Geometry check sheet. Reference: the model listing, model coordinates, mm. Face numbers are marked on the shaded views. Coordinates: 2 decimals unless noted, no trailing zeros. Write each loop counter-clockwise with the first axis right and the second up, starting at its lowest first coordinate (ties: lowest second). Pieces come first, ordered by that corner, then holes. Notation, with made-up numbers: (26, 39.25) -> (34, 39.25) arc R28 ccw to (34, 74.25) -> close; hole circle Ø9 at (36.25, 52.25). An arc over 180 degrees is marked (long way). Answer in a Markdown table with one row per item. Add a question column.
Q1. Release check for a two-part mould opening along Z. For the marked faces 1, 2 and 3 record: pulls with the +Z half, pulls with the -Z half, needs draft (parallel to the pull), parting line crosses it, or undercut.
Q2. Thickness scan on line 1 (Y direction, x = 11, z = -9.75); line 2 (Z direction, x = -8.5, y = -0.5); line 3 (X direction, y = 9.5, z = -3). Record the ranges inside material, lowest first.
Q3. Section check A-A, the plane y = 0. Record the boundary of the cut face in (x, z).
Q4. Gauge pin test, flat ends, axial feed: P1, Ø12, axis at x = 17, y = -5.5, coming from the +Z side; P2, Ø3, axis at y = -3, z = 11.5, coming from the -X side; P3, Ø2, axis at x = -17.5, y = 3, coming from the -Z side. Record the tip position at first contact, or that the pin passes through.
Q5. Section check C-C, the plane x = -15. Record the boundary of the cut face in (y, z).
Q6. Section check B-B, the plane y = 6.75. Record the boundary of the cut face in (x, z), and give its area (3 significant figures).
Q7. Section check D-D, the plane z = -5. Record the boundary of the cut face in (x, y), and give its area (3 significant figures).
```python
from build123d import *

# Parameters (mm, degrees)
F1_R   = 10.95
F1_R_2 = 10.75
F1_R_3 = 9.15
F1_R_4 = 12.55


with BuildPart() as f2:
    # F2: sweep along a path in F0
    with BuildLine(Plane.XZ) as f2_path:
        ThreePointArc((7.7781745931, 7.7781745931), (10.1626748576, 4.209517756), (11, 0))
    # F1 (on Top) → F2 (sweep)
    with BuildSketch(Plane.XY):
        with Locations((11, 0)):
            Circle(F1_R)
        with Locations((11, 0)):
            Circle(F1_R_2, mode=Mode.SUBTRACT)
        with Locations((11, 0)):
            Circle(F1_R_2)
        with Locations((11, 0)):
            Circle(F1_R_3, mode=Mode.SUBTRACT)
    sweep(path=f2_path.line)

    # F3: sweep along a path in F0
    with BuildLine(Plane.XZ) as f3_path:
        Line((11, 0), (11, -27.5))
    # F1 (on Top) → F3 (sweep)
    with BuildSketch(Plane.XY):
        with Locations((11, 0)):
            Circle(F1_R_4)
        with Locations((11, 0)):
            Circle(F1_R, mode=Mode.SUBTRACT)
        with Locations((11, 0)):
            Circle(F1_R)
        with Locations((11, 0)):
            Circle(F1_R_2, mode=Mode.SUBTRACT)
    sweep(path=f3_path.line)

    # F4: F2 across face


with BuildPart() as f2_1:
    add(f2.part)
    add(f2.part.mirror(Plane(origin=(7.7781745931, 0, 7.7781745931), x_dir=(0, -1, 0), z_dir=(-0.7071067812, 0, 0.7071067812))))


solid = f2_1.part
```
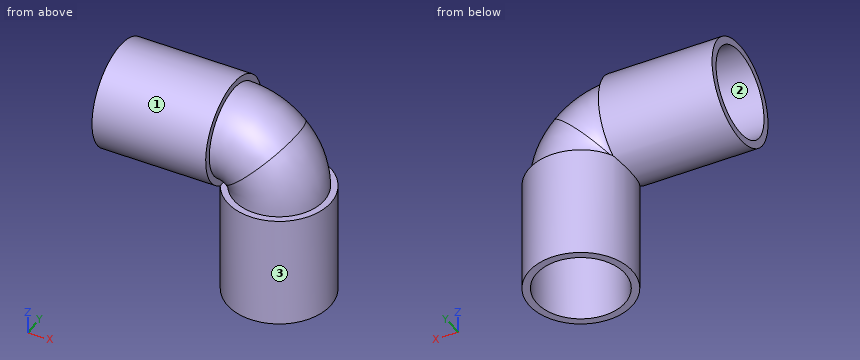
Calculated:
| question | item | result |
|---|---|---|
| 1 | face 1 | parting line crosses it |
| 1 | face 2 | undercut |
| 1 | face 3 | needs draft |
| 2 | line 1 | y = -12.55 to -10.75, 10.75 to 12.55 |
| 2 | line 2 | z = -1.54 to 0.26, 21.74 to 23.54 |
| 2 | line 3 | x = 2.8 to 5.97, 16.03 to 19.2 |
| 3 | outline | (-27.5, -1.55) -> (-1.55, -1.55) -> (-1.55, -27.5) -> (0.25, -27.5) -> (0.25, 0) -> (1.85, 0) arc R1.85 ccw to (0, 1.85) -> (0, 0.25) -> (-27.5, 0.25) -> close; (-27.5, 21.75) -> (0, 21.75) -> (0, 20.15) arc R20.15 cw to (20.15, 0) -> (21.75, 0) -> (21.75, -27.5) -> (23.55, -27.5) -> (23.55, 0) -> (21.95, 0) arc R21.95 ccw to (0, 21.95) -> (0, 23.55) -> (-27.5, 23.55) -> close; hole (0, 0) -> (0.05, 0) arc R0.05 ccw to (0, 0.05) -> close |
| 4 | P1 | stops at z = 18.18 |
| 4 | P2 | stops at x = 14.5 |
| 4 | P3 | stops at z = -1.39 |
| 5 | outline | circle Ø25.1 at (0, 11); hole circle Ø21.5 at (0, 11) |
| 6 | outline | (-27.5, 0.42) -> (0, 0.42) -> (0, 2.38) arc R2.38 cw to (2.38, 0) -> (0.42, 0) -> (0.42, -27.5) -> (2.63, -27.5) -> (2.63, 0) -> (4.82, 0) arc R4.82 ccw to (0, 4.82) -> (0, 2.63) -> (-27.5, 2.63) -> close; (-27.5, 19.37) -> (0, 19.37) -> (0, 17.18) arc R17.18 cw to (17.18, 0) -> (19.37, 0) -> (19.37, -27.5) -> (21.58, -27.5) -> (21.58, 0) -> (19.62, 0) arc R19.62 ccw to (0, 19.62) -> (0, 21.58) -> (-27.5, 21.58) -> close |
| 6 | area | 328 mm² |
| 7 | outline | circle Ø25.1 at (11, 0); hole circle Ø21.5 at (11, 0) |
| 7 | area | 132 mm² |
